Can you work these out from the model? Positions are in its coordinate system, mm. A direction names the side the tool comes from. Give positions to 0.01 mm unless a question says otherwise; leave off trailing zeros. Order: outer loops, then holes, each group sorted by start corner. A loop starts at its lowest first (then second) coordinate and runs counter-clockwise, first axis right, second up. Notation, with made-up numbers: (83.25, 0) - (121.25, 0) arc R23 cw to (121.25, 34) - close; hole circle Ø10 at (48, -20.75). An arc over 180 degrees is marked (long way). Answer as CSV lines item,"result".
Autodesk Inventor part; units mm, degrees
ref_plane "Start plane" through (0, 0, -17.5) normal (0, 0, 1) x (1, 0, 0)
ref_plane "End plane" through (0, 0, 747.5) normal (0, 0, 1) x (1, 0, 0)
ref_plane "Work Plane5" through (0, 0, 747.5) normal (0, 0, 1) x (1, 0, 0)
ref_plane "Start plane" through (0, 0, -17.5) normal (0, 0, 1) x (1, 0, 0)
ref_plane "End plane" through (0, 0, 747.5) normal (0, 0, 1) x (1, 0, 0)
sketch "Sketch" plane through (0, 0, 0) normal (0, 0, 1) x (1, 0, 0)
  line L0 (-17.5, -14.3) -> (-17.5, 14.3)
  line L1 (-14.3, 17.5) -> (14.3, 17.5)
  line L2 (17.5, 14.3) -> (17.5, -14.3)
  line L3 (14.3, -17.5) -> (-14.3, -17.5)
  arc A0 (-17.5, -14.3) -> (-14.3, -17.5) centre (-14.3, -14.3) ccw
  arc A1 (-14.3, 17.5) -> (-17.5, 14.3) centre (-14.3, 14.3) ccw
  arc A2 (17.5, 14.3) -> (14.3, 17.5) centre (14.3, 14.3) ccw
  arc A3 (14.3, -17.5) -> (17.5, -14.3) centre (14.3, -14.3) ccw
  arc A4 (-14.3, 15.9) -> (-15.9, 14.3) centre (-14.3, 14.3) ccw
  line L4 (-14.3, 15.9) -> (14.3, 15.9)
  arc A5 (15.9, 14.3) -> (14.3, 15.9) centre (14.3, 14.3) ccw
  line L5 (15.9, 14.3) -> (15.9, -14.3)
  arc A6 (14.3, -15.9) -> (15.9, -14.3) centre (14.3, -14.3) ccw
  line L6 (14.3, -15.9) -> (-14.3, -15.9)
  arc A7 (-15.9, -14.3) -> (-14.3, -15.9) centre (-14.3, -14.3) ccw
  line L7 (-15.9, -14.3) -> (-15.9, 14.3)
  line L8 (0, 25.4278) -> (0, -25.4278) construction
  line L9 (-25.4278, 0) -> (25.4278, 0) construction
  dimension "d7" = 3.2
  dimension "d10" = 35
  dimension "d11" = 35
  dimension "d12" = 1.6
  dimension "d15" = 17.5
  dimension "d16" = 17.5
extrude "Body" add sketch "Sketch" along normal up to surface (765 mm away) from surface at -17.5
sketch "Sketch3" plane through (0, 0, 0) normal (0, 0, 1) x (1, 0, 0)
  line L0 (0, 0) -> (10, 0)
ref_plane "Work Plane3" through (0, 0, 0) normal (0, -1, 0) x (1, 0, 0)
sketch "Sketch4" plane through (0, 0, 0) normal (0, -1, 0) x (1, 0, 0)
  line L0 (-2, -17.5) -> (12, -17.5)
  line L1 (-2, 747.5) -> (12, 747.5)
  dimension "d18" = 765
ref_plane "Work Plane5" through (0, 0, 747.5) normal (0, 0, 1) x (1, 0, 0)
split "Split2" plane through (0, 0, 747.5) removes the side toward (0, 0, 1)
ref_plane "Work Plane6" through (17.5, 0, 747.5) normal (-0.7071, 0, 0.7071) x (0.7071, 0, 0.7071)
split "Split3" plane through (17.5, 0, 747.5) removes the side toward (-0.7071, 0, 0.7071)
ref_plane "Work Plane9" through (17.5, 0, -17.5) normal (-0.7071, 0, -0.7071) x (-0.7071, 0, 0.7071)
split "Split6" plane through (17.5, 0, -17.5) removes the side toward (-0.7071, 0, -0.7071)
equation "\"d7\" = G_IR"
equation "\"d10\" = G_H"
equation "\"d11\" = G_W"
equation "\"d12\" = G_T"
equation "\"d15\" = 0.5 * d10"
equation "\"d16\" = 0.5 * d11"
equation "\"d3\" = G_L"
equation "\"G_W\" = 35"
equation "\"G_H\" = 35"
equation "\"G_T\" = 1.6"
equation "\"G_IR\" = 3.2"
equation "\"G_L\" = d18"
equation "\"G_OFFSET_START\" = 17.5"
equation "\"G_OFFSET_END\" = 17.5"
equation "\"d13\" = -G_OFFSET_START"
equation "\"d14\" = G_OFFSET_END + B_L"
properties part number "AS 1163 - C350L0 35x35x1.6 SHS - 765" material "Steel, Mild"
1) I want a section at B-B on y = 4. Write out the boundary of the cut face in (x, z), plus the area to 3 significant figures.
Answer block:
outline,"(-17.5, 17.5) - (-15.9, 15.9) - (-15.9, 714.1) - (-17.5, 712.5) - close; (15.9, -15.9) - (17.5, -17.5) - (17.5, 747.5) - (15.9, 745.9) - close"
area,"2,340 mm2"
2) I want a section at C-C on z = 437. Write out the boundary of the cut face in (x, y), plus the area to 3 significant figures.
Answer block:
outline,"(-17.5, -14.3) arc R3.2 ccw to (-14.3, -17.5) - (14.3, -17.5) arc R3.2 ccw to (17.5, -14.3) - (17.5, 14.3) arc R3.2 ccw to (14.3, 17.5) - (-14.3, 17.5) arc R3.2 ccw to (-17.5, 14.3) - close; hole (-15.9, -14.3) arc R1.6 ccw to (-14.3, -15.9) - (14.3, -15.9) arc R1.6 ccw to (15.9, -14.3) - (15.9, 14.3) arc R1.6 ccw to (14.3, 15.9) - (-14.3, 15.9) arc R1.6 ccw to (-15.9, 14.3) - close"
area,"207 mm2"
3) I'm going to push a flat-ended pin straight in: P1, Ø12, axis at x = 11, y = -1, coming from the +Z side. Where does the tip first touch, or does it pass through?
Answer block:
P1,"z = 747"
4) If we mould it in two halves opening along X, with no side actions, what happens to faces 1 (the flat face through (17.5, 0, 360)), 2 (the flat face through (15.9, 0, 360)), 3 (the flat face through (0, 17, 0))? For each: +X half, -X half, draft (parallel to the pull), parting line (faces both ways), or undercut.
Answer block:
face 1,"+X half"
face 2,"undercut"
face 3,"-X half"
5) Which directions (+Z, -Z, +X, -X, +Y, -Y) give clear straight access to the entire face, cutting with the end or side of a thin tool? Please do faces 4 (the flat face through (-15.9, 0, 360)), 5 (the flat face through (0, 17.5, 360)).
Answer block:
face 4,"+Z, -Z"
face 5,"+Z, -Z, +X, -X, +Y"
6) I need wall thicknesses on line 1 along X through (y, z) = (-8, 413); line 2 along Y through (x, z) = (15.5, 579.5). Which ranges of each line are inside material? Lowest first, please. Write a range as [from, to].
Answer block:
line 1,"[-17.5, -15.9], [15.9, 17.5]"
line 2,"[-17.27, -15.36], [15.36, 17.27]"
7) I want a section at A-A on x = -8. Write out the boundary of the cut face in (y, z), plus the area to 3 significant figures.
Answer block:
outline,"(-17.5, 8) - (-15.9, 8) - (-15.9, 722) - (-17.5, 722) - close; (15.9, 8) - (17.5, 8) - (17.5, 722) - (15.9, 722) - close"
area,"2,280 mm2"
